Geometry check sheet. Reference: the model listing, model coordinates, mm. A direction names the side the tool comes from. Coordinates: 2 decimals unless noted, no trailing zeros. Write each loop counter-clockwise with the first axis right and the second up, starting at its lowest first coordinate (ties: lowest second). Pieces come first, ordered by that corner, then holes. Notation, with made-up numbers: M 56,84.25 L 67,84.25 A12 cw 67,94.25 Z; hole C -37.75,66.25 d3. An arc over 180 degrees is marked long. Write each question's results on one line, items separated by ' | '.
Autodesk Inventor part; units mm, degrees
ref_plane "YZ Plane" through (0, 0, 0) normal (1, 0, 0) x (0, 1, 0)
ref_plane "XZ Plane" through (0, 0, 0) normal (0, 1, 0) x (-1, 0, 0)
ref_plane "XY Plane" through (0, 0, 0) normal (0, 0, 1) x (1, 0, 0)
sketch "Sketch1" plane through (0, 0, 0) normal (0, 1, 0) x (-1, 0, 0)
  line L0 (3.175, 0) -> (47.625, 0)
  line L1 (50.8, -3.175) -> (50.8, -73.025)
  line L2 (47.625, -76.2) -> (3.175, -76.2)
  line L3 (0, -73.025) -> (0, -3.175)
  arc A0 (50.8, -3.175) -> (47.625, 0) centre (47.625, -3.175) ccw
  arc A1 (3.175, 0) -> (0, -3.175) centre (3.175, -3.175) ccw
  arc A2 (0, -73.025) -> (3.175, -76.2) centre (3.175, -73.025) ccw
  arc A3 (47.625, -76.2) -> (50.8, -73.025) centre (47.625, -73.025) ccw
  point P0 (0, 0)
  point P1 (50.8, -76.2)
  point P2 (50.8, 0)
  point P3 (0, -76.2)
  dimension "d0" = 50.8
  dimension "d1" = 76.2
  dimension "d4" = 3.175
extrude "Extrusion1" add sketch "Sketch1" along normal blind 12.7
sketch "Sketch2" plane through (0, 12.7, 0) normal (0, 1, 0) x (1, 0, 0)
  line L0 (0, 0) -> (-6.35, 0) construction
  line L1 (-6.35, 0) -> (-6.35, 6.35) construction
  line L2 (-6.35, 6.35) -> (0, 6.35) construction
  line L3 (0, 6.35) -> (0, 0) construction
  circle A0 centre (-6.35, 6.35) radius 3.175
  line L4 (0, 3.175) -> (0, 73.025) construction
  line L5 (0, 38.1) -> (-50.8802, 38.1) construction
  line L6 (-50.8802, 38.1) -> (-25.4, 76.2) construction
  line L7 (-3.175, 76.2) -> (-47.625, 76.2) construction
  line L8 (-25.4, 76.2) -> (-25.4, 0) construction
  line L9 (-47.625, 0) -> (-3.175, 0) construction
  circle A1 centre (-6.35, 69.85) radius 3.175
  circle A2 centre (-44.45, 6.35) radius 3.175
  circle A3 centre (-44.45, 69.85) radius 3.175
  dimension "d5" = 6.35
  dimension "d6" = 6.35
  dimension "d7" = 6.35
extrude "Extrusion2" cut sketch "Sketch2" against normal through all
sketch "Sketch3" plane through (0, 12.7, 0) normal (0, 1, 0) x (1, 0, 0)
  line L0 (0, 0) -> (-12.7, 0) construction
  line L1 (0, 0) -> (12.7, 0) construction
  line L2 (-47.625, 0) -> (-3.175, 0) construction
  line L3 (-25.4, 0) -> (-25.4, 76.2) construction
  line L4 (-3.175, 76.2) -> (-47.625, 76.2) construction
  line L5 (-50.8, 0) -> (-38.1, 0) construction
  line L6 (-38.1, 0) -> (-13.2855, 0)
  line L7 (-13.2855, 0) -> (-13.2855, 76.2)
  line L8 (-13.2855, 76.2) -> (-38.1, 76.2)
  line L9 (-38.1, 76.2) -> (-38.1, 0)
  dimension "d14" = 12.7
  dimension "d15" = 180
extrude "Extrusion3" add sketch "Sketch3" along normal blind 38.1
sketch "Sketch4" plane through (0, 0, 0) normal (0, -1, 0) x (1, 0, 0)
  line L0 (0, 0) -> (-12.7, 0) construction
  line L1 (-12.7, 0) -> (-12.7, -12.7) construction
  line L2 (-12.7, -12.7) -> (0, -12.7) construction
  line L3 (0, -12.7) -> (0, 0) construction
  line L4 (-50.8, -76.2) -> (-38.1, -76.2) construction
  line L5 (-38.1, -76.2) -> (-38.1, -63.5) construction
  line L6 (-38.1, -63.5) -> (-50.8, -63.5) construction
  line L7 (-50.8, -63.5) -> (-50.8, -76.2) construction
  line L8 (-12.7, -12.7) -> (-38.1, -12.7)
  line L9 (-38.1, -12.7) -> (-38.1, -63.5)
  line L10 (-38.1, -63.5) -> (-12.7, -63.5)
  line L11 (-12.7, -63.5) -> (-12.7, -12.7)
  dimension "d18" = 12.7
  dimension "d19" = 12.7
  dimension "d20" = 12.7
  dimension "d21" = 12.7
extrude "Extrusion4" cut sketch "Sketch4" against normal blind 6.35
sketch "Sketch5" plane through (-13.2855, 12.7, 0) normal (1, 0, 0) x (0, 0, -1)
  line L0 (0, 38.1) -> (76.2, 38.1) construction
  line L1 (38.1, 38.1) -> (38.1, 0) construction
  line L2 (73.025, 0) -> (3.175, 0) construction
  line L3 (76.2, 0) -> (76.2, 38.1) construction
  line L4 (76.2, 19.05) -> (0, 19.05) construction
  circle A0 centre (38.1, 19.05) radius 6.35
  line L5 (38.1, 19.05) -> (12.7, 19.05)
  line L6 (38.1, 19.05) -> (63.5, 19.05) construction
  circle A1 centre (12.7, 19.05) radius 6.35
  circle A2 centre (63.5, 19.05) radius 6.35
  point P0 (0, -12.7)
  dimension "d24" = 12.7
  dimension "d25" = 25.4
  dimension "d26" = 180
  dimension "d27" = 12.7
extrude "Extrusion5" cut sketch "Sketch5" against normal through all
properties part number "Near Gantry Bracket"
Q1. Sectioned sample at A-A on z = -38.1. Record the cut outline in (x, y).
Geometry check:
outline: M -50.8,0 L -38.1,0 L -38.1,6.35 L -12.7,6.35 L -12.7,0 L 0,0 L 0,12.7 L -13.29,12.7 L -13.29,25.4 L -38.1,25.4 L -38.1,12.7 L -50.8,12.7 Z; M -38.1,38.1 L -13.29,38.1 L -13.29,50.8 L -38.1,50.8 Z
Q2. Access from +Z, -Z, +X, -X, +Y, -Y to the whole of each face (thin tool, end or side, straight path). Record for faces 5 (the flat face through (-42, 0, -38)), 6 (the flat face through (-38.1, 31, -47)), 7 (the flat face through (-25, 3, -12.7)).
Geometry check:
face 5: +Z, -Z, +X, -X, -Y | face 6: +Z, -Z, -X, +Y | face 7: -Y
Q3. Sectioned sample at B-B on x = -23. Record the cut outline in (y, z).
Geometry check:
outline: M 0,-76.2 L 50.8,-76.2 L 50.8,0 L 0,0 L 0,-12.7 L 6.35,-12.7 L 6.35,-63.5 L 0,-63.5 Z; hole C 31.75,-63.5 d12.7; hole C 31.75,-38.1 d12.7; hole C 31.75,-12.7 d12.7
Q4. Scan lines: probe 1 along X at (y, z) = (8, -69.85) (3 decimals); probe 2 along Z at (x, y) = (-44.45, 10) (3 decimals); probe 3 along X at (y, z) = (4, -69). Record each from-to range of solid material in increasing order.
Geometry check:
probe 1: x = -50.8 to -47.625, -41.275 to -9.525, -3.175 to 0 | probe 2: z = -76.2 to -73.025, -66.675 to -9.525, -3.175 to 0 | probe 3: x = -50.8 to -47.51, -41.39 to -9.41, -3.29 to 0
Q5. Sectioned sample at D-D on y = 21. Record the cut outline in (x, z).
Geometry check:
outline: M -38.1,-76.2 L -13.29,-76.2 L -13.29,0 L -38.1,0 Z
Q6. Mould release check, pull along Z, two halves, no side actions. Record for faces 1 (the cylindrical face through (-0.95, 6.26, -75.29)), 2 (the flat face through (-13.286, 31, -46)), 3 (the flat face through (-26, 3, -63.5)), 4 (the flat face through (-12.7, 3, -38)): pulls with the +Z half, pulls with the -Z half, needs draft (parallel to the pull), parting line crosses it, or undercut.
Geometry check:
face 1: pulls with the -Z half | face 2: needs draft | face 3: undercut | face 4: undercut
Q7. Depth check by flat-ended pin: P1, Ø1, axis at y = 19.5, z = -33.5, coming from the +X side; P2, Ø7.5, axis at x = -30, z = -39.5, coming from the -Y side; P3, Ø10, axis at x = -45, z = -31.5, coming from the +Y side; P4, Ø5.5, axis at x = -44.45, z = -69.85, coming from the +Y side. Enter the tip coordinate at first touch or a pass-through.
Geometry check:
P1: stops at x = -13.29 | P2: stops at y = 6.35 | P3: stops at y = 12.7 | P4: passes through
Q8. Sectioned sample at C-C on z = -8.5. Record the cut outline in (x, y).
Geometry check:
outline: M -50.8,0 L -46.79,0 L -46.79,12.7 L -50.8,12.7 Z; M -42.11,0 L -8.69,0 L -8.69,12.7 L -13.29,12.7 L -13.29,26.99 L -38.1,26.99 L -38.1,12.7 L -42.11,12.7 Z; M -38.1,36.51 L -13.29,36.51 L -13.29,50.8 L -38.1,50.8 Z; M -4.01,0 L 0,0 L 0,12.7 L -4.01,12.7 Z
